```python
from build123d import *
from build123d.topology import SkipClean

# Parameters (mm, degrees)
SKETCH2_W                      = 11.5
SKETCH2_H                      = 40
SKETCH3_W                      = 0.5
SKETCH3_H                      = 2
LPATTERN1_COUNT                = 7
LPATTERN1_PITCH                = 5
BOSS_EXTRUDE1_DEPTH            = 40
F_15_0_15_DIAMETER_HOLE1_D     = 15
F_15_0_15_DIAMETER_HOLE1_DEPTH = 40
F_15_0_15_DIAMETER_HOLE1_TIP   = 4.506454643
M3_CLEARANCE_HOLE1_D           = 3.4
CUT_EXTRUDE1_DEPTH             = 44.179856415
CUT_EXTRUDE1_DEPTH_BACK        = 44.179856415
SKETCH16_R                     = 1.7


with BuildPart() as part:
    # Sketch2 → Revolve1 (revolve)
    with BuildSketch(Plane.XY, mode=Mode.PRIVATE) as revolve1_sk:
        with Locations((-5.75, -20)):
            Rectangle(SKETCH2_W, SKETCH2_H)
    revolve(revolve1_sk.sketch.rotate(Axis((0, 0, 0), (0, -1, 0)), 270), axis=Axis((0, 0, 0), (0, -1, 0)))

    # Sketch3 → Cut-Revolve1 (revolve, cut)
    with BuildSketch(Plane.XY, mode=Mode.PRIVATE) as cut_revolve1_sk:
        with Locations((11.25, -36)):
            Rectangle(SKETCH3_W, SKETCH3_H)
    cut_revolve1 = revolve(cut_revolve1_sk.sketch.rotate(Axis((0, 0, 0), (0, -1, 0)), 90), axis=Axis((0, 0, 0), (0, -1, 0)), mode=Mode.SUBTRACT)

    # LPattern1: Cut-Revolve1 ×7
    with Locations(*[(0, i * LPATTERN1_PITCH, 0) for i in range(1, LPATTERN1_COUNT)]):
        add(cut_revolve1, mode=Mode.SUBTRACT)

    # Sketch6 → Boss-Extrude1 (add)
    with SkipClean():  # the faces are left unmerged after this step: merging them gives an invalid solid
        with BuildSketch(Plane(origin=(0, 0, 0), x_dir=(1, 0, 0), z_dir=(0, 1, 0))):
            with BuildLine():
                Line((-8.5, 7.745966692), (-8.5, -7.745966692))
                ThreePointArc((-8.5, -7.745966692), (0, -11.5), (8.5, -7.745966692))
                Line((8.5, -7.745966692), (8.5, 7.745966692))
                ThreePointArc((8.5, 7.745966692), (0, 11.5), (-8.5, 7.745966692))
            make_face()
        extrude(amount=BOSS_EXTRUDE1_DEPTH)

    # Ø15.0 (15) Diameter Hole1
    with Locations(Plane.XZ.offset(40)):
        with Locations((0, 0)):
            Hole(F_15_0_15_DIAMETER_HOLE1_D / 2, depth=F_15_0_15_DIAMETER_HOLE1_DEPTH)
            with Locations((0, 0, -(F_15_0_15_DIAMETER_HOLE1_DEPTH + F_15_0_15_DIAMETER_HOLE1_TIP / 2))):  # 118° drill point
                Cone(0, F_15_0_15_DIAMETER_HOLE1_D / 2, F_15_0_15_DIAMETER_HOLE1_TIP, mode=Mode.SUBTRACT)

    # M3 Clearance Hole1 (through all)
    with Locations(Plane(origin=(8.5, 0, 0), x_dir=(0, 0, -1), z_dir=(1, 0, 0))):
        with Locations((0, 8), (0, 35)):
            Hole(M3_CLEARANCE_HOLE1_D / 2)

    # Sketch16 → Cut-Extrude1 (cut, two sides: drawn at the far end of the back side and taken through both)
    with SkipClean():  # the faces are left unmerged after this step: merging them gives an invalid solid
        with BuildSketch(Plane(origin=(0, 0, 0), x_dir=(0, 0, -1), z_dir=(1, 0, 0)).offset(-CUT_EXTRUDE1_DEPTH_BACK)):
            with Locations((0, 8)):
                Circle(SKETCH16_R)
            with Locations((0, 35)):
                Circle(SKETCH16_R)
            Polygon((5.037728025, 40), (5.6954411, 18.081644681), (11.5, 18.081644681), (11.5, 40), (7.745966692, 40), align=None)
        extrude(amount=CUT_EXTRUDE1_DEPTH + CUT_EXTRUDE1_DEPTH_BACK, mode=Mode.SUBTRACT)


solid = part.part
```
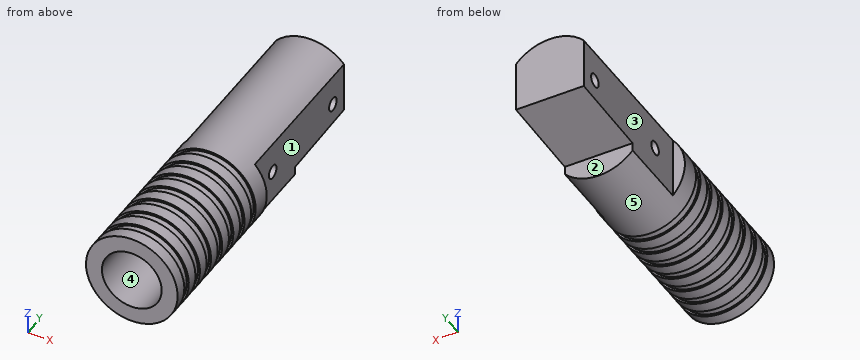
Geometry check sheet. Reference: the model listing, model coordinates, mm. Face numbers are marked on the shaded views. A direction names the side the tool comes from. Give positions to 0.01 mm unless a question says otherwise; leave off trailing zeros. Write each loop counter-clockwise with the first axis right and the second up, starting at its lowest first coordinate (ties: lowest second). Pieces come first, ordered by that corner, then holes.
1) Section check D-D, the plane y = 35. Record the boundary of the cut face in (x, z).
2) Material ranges on L1, parallel to Y at x = -4.5, z = 0; L2, parallel to X at y = -26.5, z = -0.25; L3, parallel to Y at x = -3.5, z = 0, recorded low to high.
3) Access from +Z, -Z, +X, -X, +Y, -Y to the whole of each face (thin tool, end or side, straight path). Record for the marked faces 1, 2, 3, 4 and 5.
4) Section check B-B, the plane z = 1. State how many separate pieces and enclosed holes the cut face has, and give its area (3 significant figures).
5) Gauge pin test, flat ends, axial feed: pin 1 (1 mm diameter, centred on y = -0.5, z = -3.5, fed in from +X); pin 2 (3 mm diameter, centred on x = -6, y = 9.5, fed in from +Z); pin 3 (4.5 mm diameter, centred on y = 10.5, z = 2, fed in from -X). Record the tip position at first contact, or that the pin passes through.
6) Section check A-A, the plane y = 8. Record the boundary of the cut face in (x, z), and give its area (3 significant figures).
Computed:
1. outline: (-8.5, -5.19) - (8.5, -5.19) - (8.5, -1.7) - (-8.5, -1.7) - close; (-8.5, 1.7) - (8.5, 1.7) - (8.5, 7.75) arc R11.5 ccw to (-8.5, 7.75) - close
2. L1: y = 1.8 to 6.3, 9.7 to 33.3, 36.7 to 40
2. L2: x = -11 to -7.5, 7.5 to 11
2. L3: y = 2.4 to 6.3, 9.7 to 33.3, 36.7 to 40
3. face 1: +Z, -Z, +X, +Y
3. face 2: -Z, +X, -X, +Y
3. face 3: +Z, -Z, -X, +Y
3. face 4: -Y
3. face 5: +Y, -Y
4. separate pieces: 3
4. enclosed holes: 0
4. area: 862 mm2
5. pin 1: stops at x = 11.1
5. pin 2: stops at z = 10.58
5. pin 3: stops at x = -8.5
6. outline: (-8.5, -7.75) arc R11.5 ccw to (8.5, -7.75) - (8.5, -1.7) - (-8.5, -1.7) - close; (-8.5, 1.7) - (8.5, 1.7) - (8.5, 7.75) arc R11.5 ccw to (-8.5, 7.75) - close
6. area: 294 mm2
